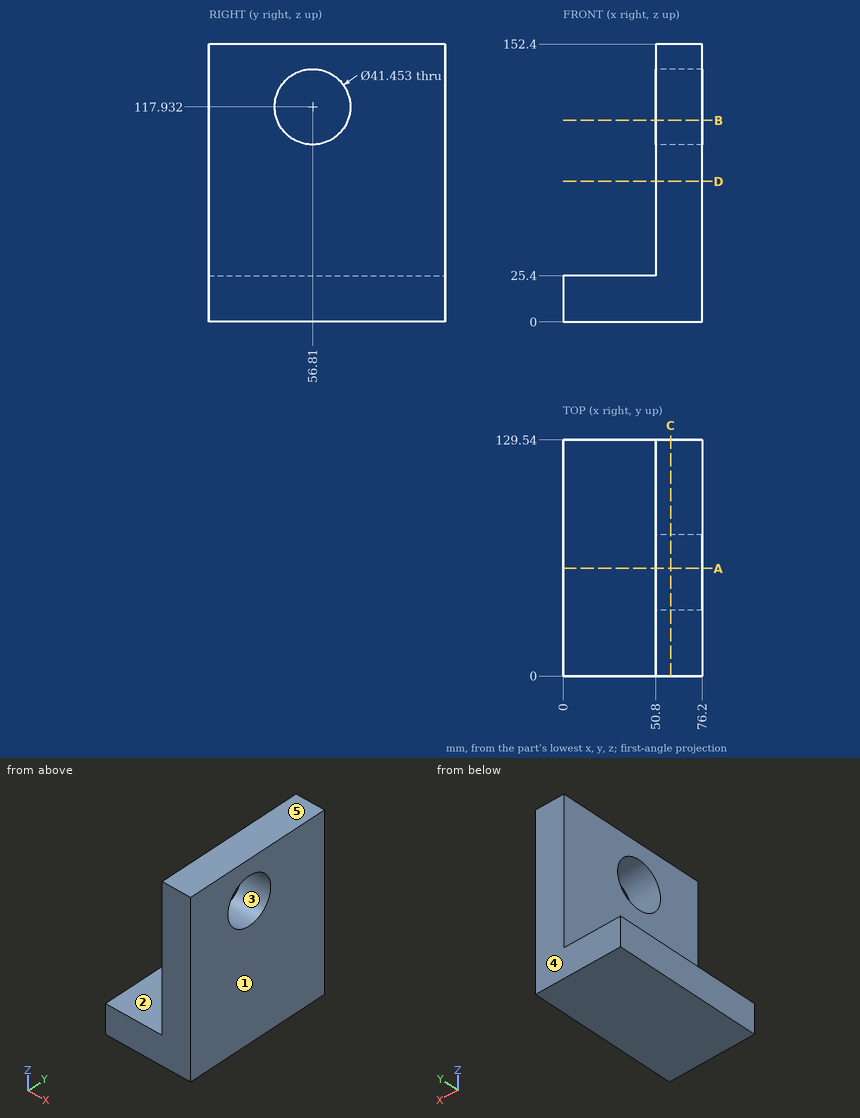
Check sheet for the drawn part. Datum: minimum x, y, z corner. Units: mm. A direction names the side the tool comes from. Round coordinates to 2 decimals unless told otherwise and drop trailing zeros. Write each loop counter-clockwise with the first axis right and the second up, starting at its lowest first coordinate (ties: lowest second). Pieces come first, ordered by that corner, then holes. Notation, with made-up numbers: (-35.75, 8.25) -> (-21.75, 8.25) arc R18 cw to (-21.75, 31.25) -> close; hole circle Ø2 at (4, 43). An arc over 180 degrees is marked (long way). Write each question's results on one line, items separated by ' | '. Start each with the question number.
1. Cross-section at C-C (x = 59). Enter the section's corners in (y, z), then the cut area to 3 significant figures.
2. Cross-section at B-B (z = 110.5). Enter the section's corners in (x, y).
3. Set-up check for the marked faces 1 and 2: record each of +Z, -Z, +X, -X, +Y, -Y from which the full face is reachable in a straight line by a thin tool's end or side.
4. Material ranges on probe 1 along Z at (x, y) = (11.5, 89); probe 2 along X at (y, z) = (119.5, 32); probe 3 along Z at (x, y) = (51, 72.5) (1 decimal), recorded low to high. Write a range as from..to.
5. Cross-section at D-D (z = 77). Enter the section's corners in (x, y), then the cut area to 3 significant figures.
6. Cross-section at A-A (y = 59). Enter the section's corners in (x, z).
7. Depth check by flat-ended pin: P1, Ø2, axis at x = 13.5, y = 13, coming from the +Z side; P2, Ø6, axis at y = 15.5, z = 66.5, coming from the -X side. Enter the tip coordinate at first touch or a pass-through.
8. Draft check along Z on the marked faces 3, 4 and 5. Enter one of: +Z half, -Z half, draft (parallel to the pull), parting line (faces both ways), or undercut.
Solutions:
1) outline: (0, 0) -> (129.54, 0) -> (129.54, 152.4) -> (0, 152.4) -> close; hole circle Ø41.45 at (56.81, 117.93) | area: 18,400 mm2
2) outline: (50.8, 0) -> (76.2, 0) -> (76.2, 37.46) -> (50.8, 37.46) -> close; (50.8, 76.16) -> (76.2, 76.16) -> (76.2, 129.54) -> (50.8, 129.54) -> close
3) face 1: +Z, -Z, +X, +Y, -Y | face 2: +Z, -X, +Y, -Y
4) probe 1: z = 0..25.4 | probe 2: x = 50.8..76.2 | probe 3: z = 0..104.4, 131.5..152.4
5) outline: (50.8, 0) -> (76.2, 0) -> (76.2, 129.54) -> (50.8, 129.54) -> close | area: 3,290 mm2
6) outline: (0, 0) -> (76.2, 0) -> (76.2, 97.32) -> (50.8, 97.32) -> (50.8, 25.4) -> (0, 25.4) -> close; (50.8, 138.54) -> (76.2, 138.54) -> (76.2, 152.4) -> (50.8, 152.4) -> close
7) P1: stops at z = 25.4 | P2: stops at x = 50.8
8) face 3: undercut | face 4: draft | face 5: +Z half
